Autodesk Inventor part; units mm, degrees
ref_plane "YZ Plane" through (0, 0, 0) normal (1, 0, 0) x (0, 1, 0)
ref_plane "XZ Plane" through (0, 0, 0) normal (0, 1, 0) x (-1, 0, 0)
ref_plane "XY Plane" through (0, 0, 0) normal (0, 0, 1) x (1, 0, 0)
sketch "Sketch1" plane through (0, 0, 0) normal (0, 1, 0) x (-1, 0, 0)
  circle A0 centre (0, 0) radius 12.1
  circle A1 centre (0, 0) radius 3.15
  circle A2 centre (0, 0) radius 1
  circle A3 centre (-8.5, 0) radius 1.5
  circle A4 centre (8.5, 0) radius 1.5
  dimension "d0" = 24.2
  dimension "d1" = 6.3
  dimension "d6" = 2
  dimension "d16" = 3
  dimension "d17" = 3
  dimension "d18" = 8.5
  dimension "d19" = 8.5
extrude "Extrusion1" add sketch "Sketch1" against normal blind 30.7 contours A0 | A1 | A2 | A3 | A4
extrude "Extrusion2" add sketch "Sketch1" along normal blind 2 contours A1 | A2
extrude "Extrusion3" add sketch "Sketch1" along normal blind 8.5 contours A2
ref_plane "Work Plane1" through (0, 3.7375, 0) normal (0, 1, 0) x (1, 0, 0)
sketch "Sketch2" plane through (0, 3.7375, 0) normal (0, 1, 0) x (1, 0, 0)
  circle A0 centre (0, 0) radius 5
  circle A1 centre (0, 0) radius 1
  circle A2 centre (0, 0) radius 4
  dimension "d10" = 10
  dimension "d11" = 8
extrude "Extrusion4" add sketch "Sketch2" along normal blind 1.5 contours A0 | A2
extrude "Extrusion5" add sketch "Sketch2" along normal blind 6 contours A2
extrude "Extrusion6" cut sketch "Sketch1" against normal blind 5 contours A3 | A4
properties part number "Motor"
Build history of the part. All positions in model axes, mm. A direction names the side the tool comes from. Give positions to 0.01 mm unless a question says otherwise; leave off trailing zeros. Loops run counter-clockwise (first coordinate to the right, second up) from the corner with the lowest first, then second, coordinate; pieces in that order, holes last. Notation, with made-up numbers: (63.5, 85) -> (116.5, 85) arc R9 cw to (116.5, 95) -> close; hole circle Ø3 at (25.25, 89). An arc over 180 degrees is marked (long way). Answer in a Markdown table with one row per item.
Item 1: Flat gauge pins, fed straight in: P1, Ø1.5, axis at y = -15, z = -3, coming from the +X side; P2, Ø5, axis at x = 8.5, z = 0, coming from the +Y side; P3, Ø1, axis at y = -7, z = 6, coming from the -X side. Where does each tip first touch, or does it go through?
Findings below:
| item | result |
|---|---|
| P1 | stops at x = 11.89 |
| P2 | stops at y = 0 |
| P3 | stops at x = -10.78 |
Item 2: Tool access for faces 4 (the flat face through (1, 9.738, 1)), 5 (the cylindrical face through (-1.08, 4.48, -4.88)), 6 (the cylindrical face through (0, 3, 1)): list every direction of +Z, -Z, +X, -X, +Y, -Y with a clear straight run to the whole face (end or side of a thin tool).
Findings below:
| item | result |
|---|---|
| face 4 | +Z, -Z, +X, -X, +Y |
| face 5 | +Y |
| face 6 | none |
Item 3: Slice it at C-C on y = -26. Write the cut outline in (x, z).
Findings below:
| item | result |
|---|---|
| outline | circle Ø24.2 at (0, 0) |
Item 4: Probe line 1 along Y through (x, z) = (2.5, 2.25); line 2 along Z through (x, y) = (0, 9.2). List the from-to ranges inside material, lowest first. Write a range as [from, to].
Findings below:
| item | result |
|---|---|
| line 1 | y = [-30.7, 0], [3.74, 9.74] |
| line 2 | z = [-4, -1], [1, 4] |
Item 5: Mould opens along Z. For faces 1 (the flat face through (-8, -5, 0)), 2 (the cylindrical face through (-11.18, -15.14, -4.63)), 3 (the flat face through (0, -30.7, 0)) say: pulls with the +Z half, pulls with the -Z half, needs draft (parallel to the pull), parting line crosses it, or undercut.
Findings below:
| item | result |
|---|---|
| face 1 | undercut |
| face 2 | parting line crosses it |
| face 3 | needs draft |
Item 6: Slice it at B-B on x = -8.5. Write the cut outline in (y, z), plus the area to 3 significant figures.
Findings below:
| item | result |
|---|---|
| outline | (-30.7, -8.61) -> (0, -8.61) -> (0, -1.5) -> (-5, -1.5) -> (-5, 1.5) -> (0, 1.5) -> (0, 8.61) -> (-30.7, 8.61) -> close |
| area | 514 mm² |
Item 7: Slice it at D-D on z = 10.25. Write the cut outline in (x, y).
Findings below:
| item | result |
|---|---|
| outline | (-6.43, -30.7) -> (6.43, -30.7) -> (6.43, 0) -> (-6.43, 0) -> close |
